Autodesk Inventor part; units mm, degrees
ref_plane "YZ Plane" through (0, 0, 0) normal (1, 0, 0) x (0, 1, 0)
ref_plane "XZ Plane" through (0, 0, 0) normal (0, 1, 0) x (-1, 0, 0)
ref_plane "XY Plane" through (0, 0, 0) normal (0, 0, 1) x (1, 0, 0)
sketch "스케치1" plane through (0, 0, 0) normal (0, 0, 1) x (1, 0, 0)
  line L0 (-20, 40) -> (0, 40)
  line L1 (0, 40) -> (0, 0)
  line L2 (0, 0) -> (-20, 0)
  line L3 (-20, 0) -> (-20, 40)
  circle A0 centre (0, 20) radius 6.25
  line L4 (0, -8) -> (0, 48)
  point P0 (0, 13.75)
  point P1 (0, 26.25)
  dimension "d0" = 20
  dimension "d1" = 40
  dimension "d2" = 12.5
  dimension "d3" = 20
extrude "돌출1" add sketch "스케치1" along normal blind 118 contours L0 L1 A0 L2 L3
sketch "스케치2" plane through (0, 0, 118) normal (0, 0, 1) x (1, 0, 0)
  line L0 (0, 40) -> (-20, 40)
  line L1 (0, 26.25) -> (0, 40)
  arc A0 (0, 26.25) -> (0, 13.75) centre (0, 20) ccw
  line L2 (0, 0) -> (0, 13.75)
  line L3 (-20, 0) -> (0, 0)
  line L4 (0, 36) -> (-16, 36)
  line L5 (-16, 36) -> (-16, 4)
  line L6 (-16, 4) -> (0, 4)
  dimension "d6" = 16
  dimension "d7" = 32
  dimension "d8" = 4
extrude "돌출2" cut sketch "스케치2" against normal blind 112
sketch "스케치4" plane through (0, 26.25, 0) normal (1, 0, 0) x (0, 0, -1)
  circle A0 centre (-3, 5.5) radius 1.8
  circle A1 centre (-3, -18) radius 1.8
  line L0 (0, -26.25) -> (0, -12.5)
  line L1 (0, -12.5) -> (-6, -12.5)
  line L2 (0, 0) -> (-6, 0)
  line L3 (0, 0) -> (0, 13.75)
  dimension "d19" = 3.6
  dimension "d20" = 3.6
  dimension "d21" = 3
  dimension "d22" = 5.5
  dimension "d23" = 5.5
  dimension "d24" = 3
extrude "돌출4" add sketch "스케치4" along normal blind 9.2
properties part number "hard_support_m"
Check sheet for the modelled part. Datum: model origin and axes. Units: mm. A direction names the side the tool comes from. Round coordinates to 2 decimals unless told otherwise and drop trailing zeros. Loops run counter-clockwise (first coordinate to the right, second up) from the corner with the lowest first, then second, coordinate; pieces in that order, holes last.
1. Sectioned sample at A-A on z = 3. Record the boundary of the cut face in (x, y), and give its area (3 significant figures).
2. Mould release check, pull along Y, two halves, no side actions. Record for faces 4 (the flat face through (9.2, 8, 3)), 5 (the flat face through (-10, 0, 58)), 6 (the flat face through (-16, 20, 63)): released by +Y, released by -Y, zero draft, split by the parting line, or undercut.
3. Sectioned sample at D-D on z = 49. Record the boundary of the cut face in (x, y).
4. Gauge pin test, flat ends, axial feed: pin 1 Ø4 at (y, z) = (5.5, 58.5) entering from +X; pin 2 Ø5 at (y, z) = (18, 52.5) entering from +X; pin 3 Ø12 at (x, y) = (5, 27.5) entering from +Z. Record the tip position at first contact, or that the pin passes through.
5. Sectioned sample at B-B on x = -4.75. Record the boundary of the cut face in (y, z).
6. Sectioned sample at C-C on y = 31.75. Record the boundary of the cut face in (x, z).
7. Scan lines: probe 1 along Y at (x, z) = (-1.5, 9.5); probe 2 along X at (y, z) = (29, 19.5); probe 3 along Z at (x, y) = (6.25, 8.5). Record each from-to range of solid material in increasing order.
8. Set-up check for faces 1 (the cylindrical face through (4.536, 30.232, 2.032)), 2 (the flat face through (-8, 36, 63)), 3 (the flat face through (-10, 40, 58)): record each of +Z, -Z, +X, -X, +Y, -Y from which the full face is reachable in a straight line by a thin tool's end or side.
Recorded:
1. outline: (-20, 0) - (0, 0) - (0, 6.45) - (9.2, 6.45) - (9.2, 10.05) - (0, 10.05) - (0, 13.75) arc R6.25 cw to (0, 26.25) - (0, 29.95) - (9.2, 29.95) - (9.2, 33.55) - (0, 33.55) - (0, 40) - (-20, 40) - close
1. area: 805 mm2
2. face 4: zero draft
2. face 5: released by -Y
2. face 6: undercut
3. outline: (-20, 0) - (0, 0) - (0, 4) - (-16, 4) - (-16, 36) - (0, 36) - (0, 40) - (-20, 40) - close
4. pin 1: stops at x = 0
4. pin 2: stops at x = -16
4. pin 3: stops at z = 6
5. outline: (0, 0) - (15.94, 0) - (15.94, 6) - (4, 6) - (4, 118) - (0, 118) - close; (24.06, 0) - (40, 0) - (40, 118) - (36, 118) - (36, 6) - (24.06, 6) - close
6. outline: (-20, 0) - (0, 0) - (0, 1.2) - (9.2, 1.2) - (9.2, 4.8) - (0, 4.8) - (0, 6) - (-16, 6) - (-16, 118) - (-20, 118) - close
7. probe 1: y = 0 to 4, 36 to 40
7. probe 2: x = -20 to -16
7. probe 3: z = 1.22 to 4.78
8. face 1: +X
8. face 2: +Z, +X
8. face 3: +Z, -Z, +X, -X, +Y
